Model file for the job. Use its own axes, mm. A direction names the side the tool comes from. Round coordinates to 2 decimals unless told otherwise and drop trailing zeros. Loops run counter-clockwise (first coordinate to the right, second up) from the corner with the lowest first, then second, coordinate; pieces in that order, holes last. Notation, with made-up numbers: (54.5, 74) - (94.5, 74) arc R12 cw to (94.5, 96) - close; hole circle Ø6 at (-33, 75.25). An arc over 180 degrees is marked (long way). Use one line per item in the form item = value.
from build123d import *

# Parameters (mm, degrees)
FILLET1_R     = 2.5
CHAMFER2_SIZE = 2.5


with BuildPart() as part:
    # Sketch1 → Revolve1 (revolve)
    with BuildSketch(Plane.XY, mode=Mode.PRIVATE) as revolve1_sk:
        Polygon((0, 0), (42.5, 0), (42.5, 5), (22.5, 5), (22.5, 5.29877748), (22.5, 65), (17.5, 65), (17.5, 22.82917197), (0, 5.32917197), align=None)
    revolve(revolve1_sk.sketch.rotate(Axis((0, 0, 0), (0, 1, 0)), 90), axis=Axis((0, 0, 0), (0, 1, 0)))

    # Fillet1
    fillet1_edges = [part.edges().sort_by_distance(p)[0] for p in [
        (0, 5, 42.5),
        (0, 5, 22.5),
    ]]
    fillet(fillet1_edges, radius=FILLET1_R)

    # Chamfer2
    chamfer2_edges = [part.edges().sort_by_distance(p)[0] for p in [
        (0, 65, 17.5),
    ]]
    chamfer(chamfer2_edges, length=CHAMFER2_SIZE)


solid = part.part
1. Tool access for faces 1 (the cylindrical face through (17.084, 42.387, 3.794)), 2 (the flat face through (-1, 0, -1)): list every direction of +Z, -Z, +X, -X, +Y, -Y with a clear straight run to the whole face (end or side of a thin tool).
Geometry check:
face_1 = +Y
face_2 = +Z, -Z, +X, -X, -Y
2. Flat gauge pins, fed straight in: pin 1 (4 mm diameter, centred on y = 51, z = -17.5, fed in from +X); pin 2 (1 mm diameter, centred on y = 47.5, z = 10, fed in from +X); pin 3 (2 mm diameter, centred on y = 28, z = 20.5, fed in from -X) (3 decimals); pin 4 (4 mm diameter, centred on x = -25.5, y = 49, fed in from -Z) (1 decimal). Where does each tip first touch, or does it go through?
Geometry check:
pin_1 = 16.31
pin_2 = 20.4
pin_3 = -11.225
pin_4 = through
3. Cut at A-A, the plane y = 31.5. Give the cut face in (x, z).
Geometry check:
outline = circle Ø45 at (0, 0); hole circle Ø35 at (0, 0)
4. Pull direction Z, two halves, no side cores. Call faces 3 (the conical face through (10.722, 62.621, 13.984)), 4 (the flat face through (1.6, 65, 20.1)), 5 (the cylindrical face through (-12.766, 1.268, -40.537)): +Z half, -Z half, draft (parallel to the pull), parting line (faces both ways), or undercut.
Geometry check:
face_3 = undercut
face_4 = draft
face_5 = parting line
5. Wall check: probe 1 along X at (y, z) = (34.5, 0); probe 2 along Y at (x, z) = (-33, 23); probe 3 along X at (y, z) = (10, -3). Give the ranges that are in metal, low to high.
Geometry check:
probe_1 = -22.5 to -17.5, 17.5 to 22.5
probe_2 = 0 to 4.99
probe_3 = -22.3 to -3.58, 3.58 to 22.3
